```python
from build123d import *

# Parameters (mm, degrees)
CROQUIS1_W              = 180
CROQUIS1_H              = 170
SALIENTE_EXTRUIR1_DEPTH = 90
CROQUIS2_R              = 49
CORTAR_EXTRUIR1_DEPTH   = 1
CORTAR_EXTRUIR2_START   = -1
CROQUIS3_R              = 49
CORTAR_EXTRUIR2_DEPTH   = 1
VACIADO1_START          = -89
VACIADO1_OUTLINE_W      = 168
VACIADO1_OUTLINE_H      = 178
VACIADO1_DEPTH          = 178


# Read off the part's stored shape, not the designer's step: Vaciado1
with BuildPart() as part:
    # Croquis1 → Saliente-Extruir1 (new, symmetric)
    with BuildSketch(Plane.XY):
        Rectangle(CROQUIS1_W, CROQUIS1_H)
    extrude(amount=SALIENTE_EXTRUIR1_DEPTH, both=True)

    # Croquis2 → Cortar-Extruir1 (cut)
    with BuildSketch(Plane.ZY.offset(90)):
        Circle(CROQUIS2_R)
    extrude(amount=-CORTAR_EXTRUIR1_DEPTH, mode=Mode.SUBTRACT)

    # Croquis3 → Cortar-Extruir2 (cut)
    with BuildSketch(Plane(origin=(90, 0, 0), x_dir=(0, 0, -1), z_dir=(1, 0, 0)).offset(CORTAR_EXTRUIR2_START)):
        with Locations(Location((0, 0, 0), (0, 0, 180))):
            Circle(CROQUIS3_R)
    extrude(amount=CORTAR_EXTRUIR2_DEPTH, mode=Mode.SUBTRACT)

    # Vaciado1 outline → Vaciado1 (cut)
    with BuildSketch(Plane.YZ.offset(VACIADO1_START)):
        Rectangle(VACIADO1_OUTLINE_W, VACIADO1_OUTLINE_H)
    extrude(amount=VACIADO1_DEPTH, mode=Mode.SUBTRACT)


solid = part.part
```
Input: part model. Units: mm. Frame: model coordinates. A direction names the side the tool comes from. Give positions to 0.01 mm unless a question says otherwise; leave off trailing zeros. Order: outer loops, then holes, each group sorted by start corner. A loop starts at its lowest first (then second) coordinate and runs counter-clockwise, first axis right, second up. Notation, with made-up numbers: (14.5, 27.25) - (66.5, 27.25) arc R19 ccw to (66.5, 47.25) - close; hole circle Ø7 at (-18.5, -21). An arc over 180 degrees is marked (long way). Put each result on its own line as item: value.
Item 1: Section query A-A, the plane z = 0. Return loops of the section in (x, y).
Found:
outline: (-90, -85) - (90, -85) - (90, -49) - (89, -49) - (89, -84) - (-89, -84) - (-89, -49) - (-90, -49) - close; (-90, 49) - (-89, 49) - (-89, 84) - (89, 84) - (89, 49) - (90, 49) - (90, 85) - (-90, 85) - close
Item 2: Draft query along Z for faces 3 (the flat face through (-1, 1, -90)), 4 (the flat face through (-1, -85, 1)), 5 (the flat face through (-1, -1, 89)). Return one class per face: +Z half, -Z half, draft (parallel to the pull), parting line (faces both ways), or undercut.
Found:
face 3: -Z half
face 4: draft
face 5: undercut
Item 3: Section query D-D, the plane y = 67. Return loops of the section in (x, z).
Found:
outline: (-90, -90) - (90, -90) - (90, 90) - (-90, 90) - close; hole (-89, -89) - (89, -89) - (89, 89) - (-89, 89) - close
Item 4: Section query B-B, the plane x = -47.5. Return loops of the section in (y, z).
Found:
outline: (-85, -90) - (85, -90) - (85, 90) - (-85, 90) - close; hole (-84, -89) - (84, -89) - (84, 89) - (-84, 89) - close
Item 5: Access query for faces 1 (the flat face through (-1, 85, 1)), 2 (the flat face through (89, -39, -38)). Directions: +Z, -Z, +X, -X, +Y, -Y. A direction counts if a zero-diameter tool reaches every point of the face in a straight line with its end or side. Return the directions, or none.
Found:
face 1: +Z, -Z, +X, -X, +Y
face 2: none
Item 6: Ray query, L1, parallel to X at y = -60.5, z = -1.5; L2, parallel to Y at x = -9, z = 29; L3, parallel to Y at x = -89.3, z = 0. Return the intervals inside material, ascending. Write a range as from..to.
Found:
L1: x = -90..-89, 89..90
L2: y = -85..-84, 84..85
L3: y = -85..-49, 49..85
Item 7: Section query C-C, the plane y = 0. Return loops of the section in (x, z).
Found:
outline: (-90, -90) - (90, -90) - (90, -49) - (89, -49) - (89, -89) - (-89, -89) - (-89, -49) - (-90, -49) - close; (-90, 49) - (-89, 49) - (-89, 89) - (89, 89) - (89, 49) - (90, 49) - (90, 90) - (-90, 90) - close
